from build123d import *

# Parameters (mm, degrees)
SKETCH1_W           = 12.7
SKETCH1_H           = 12.7
BOSS_EXTRUDE1_DEPTH = 2.54
FILLET1_R           = 0.635
SHELL1_START        = 0.635
SHELL1_OUTLINE_W    = 1.905
SHELL1_OUTLINE_H    = 11.43
SHELL1_DEPTH        = 11.43
SKETCH2_R           = 2.54
BOSS_EXTRUDE2_DEPTH = 1.905
BOSS_EXTRUDE3_DEPTH = 0.00254


# Read off the part's stored shape, not the designer's step: Shell1
with BuildPart() as part:
    # Sketch1 → Boss-Extrude1 (new body)
    with BuildSketch(Plane(origin=(0, 0, 0), x_dir=(1, 0, 0), z_dir=(0, 1, 0))):
        with Locations((6.35, 6.35)):
            Rectangle(SKETCH1_W, SKETCH1_H)
    extrude(amount=BOSS_EXTRUDE1_DEPTH)

    # Fillet1
    fillet1_edges = [part.edges().sort_by_distance(p)[0] for p in [
        (0, 1.27, -12.7),
        (12.7, 1.27, -12.7),
        (12.7, 1.27, 0),
        (0, 1.27, 0),
    ]]
    fillet(fillet1_edges, radius=FILLET1_R)

    # Shell1 outline → Shell1 (cut)
    with BuildSketch(Plane.YZ.offset(SHELL1_START)):
        with Locations((0.9525, -6.35)):
            Rectangle(SHELL1_OUTLINE_W, SHELL1_OUTLINE_H)
    extrude(amount=SHELL1_DEPTH, mode=Mode.SUBTRACT)

    # Sketch2 → Boss-Extrude2 (add)
    with BuildSketch(Plane(origin=(0, 1.905, 0), x_dir=(-1, 0, 0), z_dir=(0, -1, 0))):
        with Locations(Location((-6.35, 6.35, 0), (0, 0, 270))):
            Circle(SKETCH2_R)
    extrude(amount=BOSS_EXTRUDE2_DEPTH)

    # Sketch3 → Boss-Extrude3 (add)
    with BuildSketch(Plane(origin=(0, 2.54, 0), x_dir=(1, 0, 0), z_dir=(0, 1, 0))):
        with BuildLine():
            add(Edge.make_bspline(
                [(6.432224359, 9.726897436), (6.455251183, 9.725706594), (6.500646544, 9.723358955), (6.565830657, 9.703776202), (6.625237948, 9.670782167), (6.67786071, 9.626551956), (6.722312309, 9.573817503), (6.754934047, 9.513997076), (6.774770917, 9.4485002), (6.777054423, 9.402877937), (6.778217949, 9.379631811)],
                knots=[0, 0, 0, 0, 1.013817282, 1.998651736, 2.969187861, 3.991244904, 5.013301947, 5.9920405, 6.976874954, 8, 8, 8, 8], degree=3))
            add(Edge.make_bspline(
                [(6.778217949, 9.379631811), (6.777069623, 9.356799998), (6.774815935, 9.311990578), (6.754640219, 9.247480223), (6.72234006, 9.18798217), (6.677853125, 9.135257928), (6.625239865, 9.091024972), (6.565830149, 9.058031637), (6.500646676, 9.038448699), (6.455251227, 9.036101085), (6.432224359, 9.034910256)],
                knots=[0, 0, 0, 0, 1.009116963, 1.980479832, 2.963706907, 3.990451133, 5.017195359, 5.992182391, 6.981533323, 8, 8, 8, 8], degree=3))
            add(Edge.make_bspline(
                [(6.432224359, 9.034910256), (6.409185604, 9.036078537), (6.363766721, 9.0383817), (6.298671705, 9.058314456), (6.238667642, 9.090077481), (6.186076647, 9.134036199), (6.141182927, 9.18595953), (6.109829566, 9.245948014), (6.089538882, 9.310915397), (6.087350713, 9.356368241), (6.086230769, 9.379631811)],
                knots=[0, 0, 0, 0, 1.016706445, 2.004347467, 2.981433789, 4.000427929, 5.018214116, 5.995300439, 6.973959266, 8, 8, 8, 8], degree=3))
            add(Edge.make_bspline(
                [(6.086230769, 9.379631811), (6.087378792, 9.402886411), (6.089631872, 9.448525304), (6.109660198, 9.513804333), (6.141367354, 9.574006456), (6.186018885, 9.626497828), (6.238654577, 9.671002499), (6.29850054, 9.703611102), (6.363785957, 9.723387734), (6.409192077, 9.72571628), (6.432224359, 9.726897436)],
                knots=[0, 0, 0, 0, 1.022642663, 2.007012786, 2.980863166, 4.002438329, 5.024013493, 6.00229059, 6.986660713, 8, 8, 8, 8], degree=3))
        make_face()
        with BuildLine():
            add(Edge.make_bspline(
                [(6.432224359, 8.017282051), (6.455229408, 8.01602074), (6.500522375, 8.013537435), (6.565964538, 7.995004793), (6.625026467, 7.96170826), (6.677835723, 7.918278705), (6.722489899, 7.866027151), (6.754764929, 7.806440642), (6.774863399, 7.741250637), (6.777082284, 7.695815172), (6.778217949, 7.672560497)],
                knots=[0, 0, 0, 0, 1.016957001, 2.002212695, 2.9757545, 3.99499976, 5.013036768, 5.994806404, 6.97370641, 8, 8, 8, 8], degree=3))
            add(Edge.make_bspline(
                [(6.778217949, 7.672560497), (6.777089724, 7.649302087), (6.774885374, 7.603859325), (6.754625849, 7.538542292), (6.722538129, 7.478466037), (6.67783214, 7.425654573), (6.625245168, 7.381406547), (6.565828744, 7.348417057), (6.500647041, 7.328833105), (6.45525135, 7.32648563), (6.432224359, 7.325294872)],
                knots=[0, 0, 0, 0, 1.023218912, 1.999186227, 2.986238111, 4.008388923, 5.030539734, 6.0011649, 6.986089706, 8, 8, 8, 8], degree=3))
            add(Edge.make_bspline(
                [(6.432224359, 7.325294872), (6.409191911, 7.326475947), (6.363785464, 7.328804333), (6.298502441, 7.348582131), (6.238647359, 7.381186296), (6.186047174, 7.425708246), (6.141141459, 7.478279027), (6.109966022, 7.538731843), (6.089517785, 7.603834699), (6.087343571, 7.64929375), (6.086230769, 7.672560497)],
                knots=[0, 0, 0, 0, 1.013427518, 1.99788335, 2.976245624, 3.997909735, 5.019573847, 6.001765691, 6.977268297, 8, 8, 8, 8], degree=3))
            add(Edge.make_bspline(
                [(6.086230769, 7.672560497), (6.087350912, 7.695823654), (6.089539471, 7.741275691), (6.109827339, 7.806248907), (6.141191423, 7.866215177), (6.186043429, 7.91822492), (6.238867187, 7.961926791), (6.298365885, 7.994841981), (6.363910067, 8.01356642), (6.409213828, 8.016030503), (6.432224359, 8.017282051)],
                knots=[0, 0, 0, 0, 1.025808215, 2.00424526, 2.981110158, 3.998665696, 5.017428914, 5.998734231, 6.983523959, 8, 8, 8, 8], degree=3))
        make_face()
        with BuildLine():
            add(Edge.make_bspline(
                [(6.432224359, 5.408897436), (6.455251183, 5.407706594), (6.500646544, 5.405358955), (6.565830657, 5.385776202), (6.625237948, 5.352782167), (6.67786071, 5.308551956), (6.722312309, 5.255817503), (6.754934047, 5.195997076), (6.774770917, 5.1305002), (6.777054423, 5.084877937), (6.778217949, 5.061631811)],
                knots=[0, 0, 0, 0, 1.013817282, 1.998651736, 2.969187861, 3.991244904, 5.013301947, 5.9920405, 6.976874954, 8, 8, 8, 8], degree=3))
            add(Edge.make_bspline(
                [(6.778217949, 5.061631811), (6.777082486, 5.038376721), (6.774863996, 4.992940445), (6.754762665, 4.92775631), (6.722498561, 4.868147384), (6.677802035, 4.815982727), (6.625228174, 4.772296035), (6.56565729, 4.740149638), (6.500666175, 4.720410262), (6.45525779, 4.718088149), (6.432224359, 4.716910256)],
                knots=[0, 0, 0, 0, 1.02653117, 2.005657786, 2.987654694, 4.005927372, 5.02540858, 5.994694477, 6.98280758, 8, 8, 8, 8], degree=3))
            add(Edge.make_bspline(
                [(6.432224359, 4.716910256), (6.409185604, 4.718078537), (6.363766721, 4.7203817), (6.298671705, 4.740314456), (6.238667642, 4.772077481), (6.186076647, 4.816036199), (6.141182927, 4.86795953), (6.109829566, 4.927948014), (6.089538882, 4.992915397), (6.087350713, 5.038368241), (6.086230769, 5.061631811)],
                knots=[0, 0, 0, 0, 1.016706445, 2.004347467, 2.981433789, 4.000427929, 5.018214116, 5.995300439, 6.973959266, 8, 8, 8, 8], degree=3))
            add(Edge.make_bspline(
                [(6.086230769, 5.061631811), (6.087378792, 5.084886411), (6.089631872, 5.130525304), (6.109660198, 5.195804333), (6.141367354, 5.256006456), (6.186018885, 5.308497828), (6.238654577, 5.353002499), (6.29850054, 5.385611102), (6.363785957, 5.405387734), (6.409192077, 5.40771628), (6.432224359, 5.408897436)],
                knots=[0, 0, 0, 0, 1.022642663, 2.007012786, 2.980863166, 4.002438329, 5.024013493, 6.00229059, 6.986660713, 8, 8, 8, 8], degree=3))
        make_face()
        Polygon((6.411871795, 3.636952324), (6.818923077, 3.422614383), (6.30056871, 2.518833333), (6.010544671, 2.660665264), align=None)
    extrude(amount=BOSS_EXTRUDE3_DEPTH)


solid = part.part
For this review, take the finished solid that the model builds, in its own axes (mm). A direction names the side the tool comes from. Round coordinates to 2 decimals unless told otherwise and drop trailing zeros. Loops run counter-clockwise (first coordinate to the right, second up) from the corner with the lowest first, then second, coordinate; pieces in that order, holes last. Notation, with made-up numbers: (5, -28.75) - (28, -28.75) arc R19 cw to (28, 5.25) - close; hole circle Ø9 at (-19, 47). An arc over 180 degrees is marked (long way). Use one line per item in the form item = value.
Item 1: Mouldability with a two-part tool opening along X and no side actions: class faces 3 (the flat face through (6, 2.54, -6)), 4 (the flat face through (6, 1, -12.065)), 5 (the flat face through (0.635, 1, -6)), 6 (the flat face through (0, 1, -6)) as +X half, -X half, draft (parallel to the pull), parting line (faces both ways), or undercut.
Answers:
face_3 = draft
face_4 = undercut
face_5 = undercut
face_6 = -X half
Item 2: Consider section C-C on x = 11.75. Write out the cut boundary in (y, z) (3 decimals), then the cut area to 3 significant figures.
Answers:
outline = (0, -12.7) - (2.54, -12.7) - (2.54, 0) - (0, 0) - (0, -0.635) - (1.905, -0.635) - (1.905, -12.065) - (0, -12.065) - close
area = 10.5 mm^2
Item 3: Consider section A-A on y = 0.95. Write out the cut boundary in (x, z) (3 decimals), then the cut area to 3 significant figures.
Answers:
outline = (0, -12.065) arc R0.635 ccw to (0.635, -12.7) - (12.065, -12.7) arc R0.635 ccw to (12.7, -12.065) - (12.7, -0.635) arc R0.635 ccw to (12.065, 0) - (0.635, 0) arc R0.635 ccw to (0, -0.635) - close; circle Ø5.08 at (6.35, -6.35); hole (0.635, -12.065) - (12.065, -12.065) - (12.065, -0.635) - (0.635, -0.635) - close
area = 50.6 mm^2
Item 4: For line 1 (X direction, y = 0.8, z = -6.25) (3 decimals); line 2 (Z direction, x = 6.5, y = 0.35) (3 decimals); line 3 (Z direction, x = 9.5, y = 0.5) (3 decimals), list the stretches that pass through material, from the lowest coordinate up.
Answers:
line_1 = 0 to 0.635, 3.812 to 8.888, 12.065 to 12.7
line_2 = -12.7 to -12.065, -8.886 to -3.814, -0.635 to 0
line_3 = -12.7 to -12.065, -0.635 to 0
Item 5: Consider section B-B on z = -1. Write out the cut boundary in (x, y) (3 decimals), then the cut area to 3 significant figures.
Answers:
outline = (0, 0) - (0.635, 0) - (0.635, 1.905) - (12.065, 1.905) - (12.065, 0) - (12.7, 0) - (12.7, 2.54) - (0, 2.54) - close
area = 10.5 mm^2
Item 6: Clearance check with a flat-ended pin moving along its axis: P1, Ø4, axis at x = 9, z = -4, coming from the +Y side. State where the tip first meets the part, or that it passes through.
Answers:
P1 = 2.54
Item 7: Tool access review of faces 1 (the flat face through (6.4, 2.543, -3.1)), 2 (the flat face through (5, 1.905, -9)): name each direction out of +Z, -Z, +X, -X, +Y, -Y from which nothing blocks a thin tool from reaching the whole face with its end or side.
Answers:
face_1 = +Z, -Z, +X, -X, +Y
face_2 = -Y
Item 8: Consider section D-D on z = -6.35. Write out the cut boundary in (x, y) (3 decimals).
Answers:
outline = (0, 0) - (0.635, 0) - (0.635, 1.905) - (3.81, 1.905) - (3.81, 0) - (8.89, 0) - (8.89, 1.905) - (12.065, 1.905) - (12.065, 0) - (12.7, 0) - (12.7, 2.54) - (0, 2.54) - close
